Read the model definition and answer for the solid it produces. Units are mm, in the model's axes. A direction names the side the tool comes from. Coordinates: 2 decimals unless noted, no trailing zeros. Write each loop counter-clockwise with the first axis right and the second up, starting at its lowest first coordinate (ties: lowest second). Pieces come first, ordered by that corner, then holes. Notation, with made-up numbers: (51, 31) -> (62, 31) arc R18 ccw to (62, 61) -> close; hole circle Ø3 at (50, 70). An arc over 180 degrees is marked (long way). Return JSON: item names as keys, results as strings.
from build123d import *

# Parameters (mm, degrees)
BOSS_EXTRUDE1_DEPTH = 1.524
FILLET1_R           = 1.524


with BuildPart() as part:
    # Sketch1 → Boss-Extrude1 (new body)
    with BuildSketch(Plane.XY):
        Polygon((0, 73.143262765), (1.524, 73.143262765), (1.524, 68.978612676), (10.474816324, 75.179605793), (7.183025054, 77.303792749), (8.009350184, 78.584324974), (6.728817959, 79.410650105), (5.902492829, 78.13011788), (-3.0948828, 83.93610811), (-2.26855767, 85.216640335), (-3.549089895, 86.042965466), (-4.375415025, 84.762433241), (-10.628767588, 88.797710347), (0, 68.978612676), align=None)
    extrude(amount=BOSS_EXTRUDE1_DEPTH)

    # Fillet1
    fillet1_edges = [part.edges().sort_by_distance(p)[0] for p in [
        (-10.628767588, 88.797710347, 0.762),
    ]]
    fillet(fillet1_edges, radius=FILLET1_R)


solid = part.part
1. The part is cut by section B-B (y = 70). Determine the outline of the cut face in (x, z), then the cut area to 3 significant figures.
Taken from the geometry:
{"outline": "(-0.55, 0) -> (0, 0) -> (0, 1.52) -> (-0.55, 1.52) -> close; (1.52, 0) -> (3, 0) -> (3, 1.52) -> (1.52, 1.52) -> close", "area": "3.08 mm2"}
2. Consider L1, parallel to Y at x = -2.75, z = 1.3; L2, parallel to X at y = 84.5, z = 0.5; L3, parallel to X at y = 82.75, z = 0.3. Determine where each line is inside the solid, lowest interval first.
Taken from the geometry:
{"L1": "y = 74.11 to 83.71, 84.47 to 85.53", "L2": "x = -8.01 to -2.73", "L3": "x = -7.39 to -1.26"}
3. The part is cut by section A-A (z = 0.8). Determine the outline of the cut face in (x, y).
Taken from the geometry:
{"outline": "(-7.84, 83.6) -> (0, 68.98) -> (0, 73.14) -> (1.52, 73.14) -> (1.52, 68.98) -> (10.47, 75.18) -> (7.18, 77.3) -> (8.01, 78.58) -> (6.73, 79.41) -> (5.9, 78.13) -> (-3.09, 83.94) -> (-2.27, 85.22) -> (-3.55, 86.04) -> (-4.38, 84.76) -> (-5.67, 85.6) arc R1.52 ccw to start"}
4. For a pull along X with two mould halves and no side action, classify faces 5 (the face through (5.94, 72.04, 0.75)), 6 (the face through (6.32, 78.78, 0.75)), 7 (the face through (1, 73.143, 1)), 8 (the face through (-3.975, 76.39, 0.751)) as +X half, -X half, draft (parallel to the pull), parting line (faces both ways), or undercut.
Taken from the geometry:
{"face 5": "+X half", "face 6": "undercut", "face 7": "undercut", "face 8": "-X half"}
5. A tool of negligible diameter and unlimited length cuts with its end or side. For faces 1 (the face through (7.59, 77.935, 0.751)), 2 (the face through (1, 78, 1.524)), 3 (the face through (1.524, 71, 1)), 4 (the face through (-5.01, 85.17, 0.75)), from which of +Z, -Z, +X, -X, +Y, -Y can it reach the whole face along a straight path? Write none if from no direction.
Taken from the geometry:
{"face 1": "+Z, -Z, +X", "face 2": "+Z, +X, -X, +Y, -Y", "face 3": "+Z, -Z, -Y", "face 4": "+Z, -Z, +Y"}
6. The part is cut by section D-D (y = 76.75). Determine the outline of the cut face in (x, z).
Taken from the geometry:
{"outline": "(-4.17, 0) -> (8.04, 0) -> (8.04, 1.52) -> (-4.17, 1.52) -> close"}
7. Flat-ended cylindrical pins translate along their axes: pin 1 Ø0.8 at (y, z) = (71.5, 0.5) entering from -X; pin 2 Ø0.5 at (x, z) = (1, 1) entering from -Y. Find the tip coordinate at first contact, or state that the pin passes through.
Taken from the geometry:
{"pin 1": "stops at x = -1.57", "pin 2": "stops at y = 73.14"}
8. The part is cut by section C-C (x = 8.25). Determine the outline of the cut face in (y, z).
Taken from the geometry:
{"outline": "(73.64, 0) -> (76.62, 0) -> (76.62, 1.52) -> (73.64, 1.52) -> close"}
